from build123d import *

# Parameters (mm, degrees)
F1_DEPTH = 12.7
F2_DEPTH = 6.35
F4_DEPTH = 25.4
F5_DEPTH = 25.4


with BuildPart() as f1:
    # F0 (on Front) → F1 (new body)
    with BuildSketch(Plane.XZ):
        with BuildLine():
            ThreePointArc((38.1, 57.15), (36.240128, 61.640128), (31.75, 63.5))
            Line((31.75, 63.5), (-31.75, 63.5))
            ThreePointArc((-31.75, 63.5), (-36.240128, 61.640128), (-38.1, 57.15))
            Line((-38.1, 57.15), (-38.1, -57.15))
            ThreePointArc((-38.1, -57.15), (-36.240128, -61.640128), (-31.75, -63.5))
            Line((-31.75, -63.5), (31.75, -63.5))
            ThreePointArc((31.75, -63.5), (36.240128, -61.640128), (38.1, -57.15))
            Line((38.1, -57.15), (38.1, 57.15))
        make_face()
        Polygon((22.86, 50.8), (25.4, 50.8), (25.4, 27.760267), (25.4, 23.039733), (25.4, 0), (25.4, -50.8), (-25.4, -50.8), (-25.4, 0), (-25.4, 23.039733), (-25.4, 27.760267), (-25.4, 50.8), (-22.86, 50.8), (-20.32, 50.8), (-17.78, 50.8), (-15.24, 50.8), (-12.7, 50.8), (-10.16, 50.8), (-7.62, 50.8), (-5.08, 50.8), (-2.54, 50.8), (0, 50.8), (2.54, 50.8), (5.08, 50.8), (7.62, 50.8), (10.16, 50.8), (12.7, 50.8), (15.24, 50.8), (17.78, 50.8), (20.32, 50.8), align=None, mode=Mode.SUBTRACT)
    extrude(amount=F1_DEPTH)

    # F0 (on Front) → F2 (join)
    with BuildSketch(Plane.XZ):
        Polygon((22.86, 27.760267), (22.86, 50.8), (20.32, 50.8), (20.32, 27.760267), (17.78, 27.760267), (17.78, 50.8), (15.24, 50.8), (15.24, 27.760267), (12.7, 27.760267), (12.7, 50.8), (10.16, 50.8), (10.16, 27.760267), (7.62, 27.760267), (7.62, 50.8), (5.08, 50.8), (5.08, 27.760267), (2.54, 27.760267), (2.54, 50.8), (0, 50.8), (-2.54, 50.8), (-2.54, 27.760267), (-5.08, 27.760267), (-5.08, 50.8), (-7.62, 50.8), (-7.62, 27.760267), (-10.16, 27.760267), (-10.16, 50.8), (-12.7, 50.8), (-12.7, 27.760267), (-15.24, 27.760267), (-15.24, 50.8), (-17.78, 50.8), (-17.78, 27.760267), (-20.32, 27.760267), (-20.32, 50.8), (-22.86, 50.8), (-22.86, 27.760267), (-25.4, 27.760267), (-25.4, 23.039733), (-22.86, 23.039733), (-22.86, 0), (-20.32, 0), (-20.32, 23.039733), (-17.78, 23.039733), (-17.78, 0), (-15.24, 0), (-15.24, 23.039733), (-12.7, 23.039733), (-12.7, 0), (-10.16, 0), (-10.16, 23.039733), (-7.62, 23.039733), (-7.62, 0), (-5.08, 0), (-5.08, 23.039733), (-2.54, 23.039733), (-2.54, 0), (0, 0), (2.54, 0), (2.54, 23.039733), (5.08, 23.039733), (5.08, 0), (7.62, 0), (7.62, 23.039733), (10.16, 23.039733), (10.16, 0), (12.7, 0), (12.7, 23.039733), (15.24, 23.039733), (15.24, 0), (17.78, 0), (17.78, 23.039733), (20.32, 23.039733), (20.32, 0), (22.86, 0), (22.86, 23.039733), (25.4, 23.039733), (25.4, 27.760267), align=None)
    extrude(amount=F2_DEPTH)

    # F3 (on Right) → F4 (join, through all)
    with BuildSketch(Plane.YZ):
        Polygon((0, -50.8), (0, 0), (-6.35, 0), (-12.7, -50.8), align=None)
    extrude(amount=F4_DEPTH)

    # F4_face (on face) → F5 (join, through all)
    with BuildSketch(Plane(origin=(0, -4.938889, -28.222222), x_dir=(0, 1, 0), z_dir=(-1, 0, 0))):
        Polygon((4.938889, -28.222222), (4.938889, 22.577778), (-7.761111, 22.577778), (-1.411111, -28.222222), align=None)
    extrude(amount=F5_DEPTH)


solid = f1.part
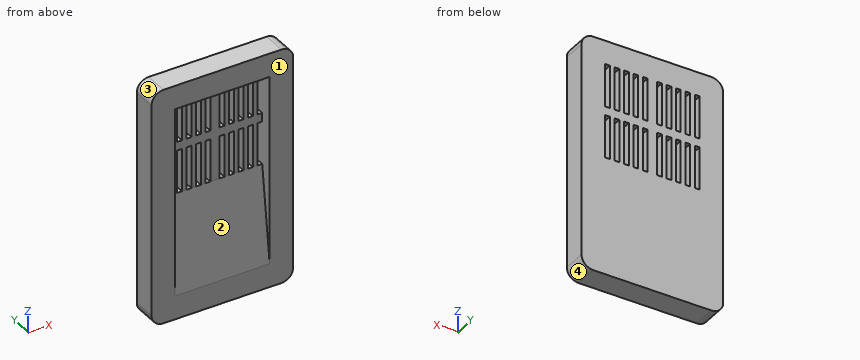
Read the model definition and answer for the solid it produces. Units are mm, in the model's axes. Face numbers are marked on the shaded views. Give positions to 0.01 mm unless a question says otherwise; leave off trailing zeros. Loops run counter-clockwise (first coordinate to the right, second up) from the corner with the lowest first, then second, coordinate; pieces in that order, holes last. Notation, with made-up numbers: (59.5, 13) -> (69.5, 13) arc R34 ccw to (69.5, 47) -> close; hole circle Ø1 at (25, 38). An arc over 180 degrees is marked (long way). Use a Markdown table: item, result.
Q1. Determine the mould class of the marked faces 1, 2, 3 and 4 for opening direction X: pulls with the +X half, pulls with the -X half, needs draft (parallel to the pull), parting line crosses it, or undercut.
Solved:
| item | result |
|---|---|
| face 1 | needs draft |
| face 2 | undercut |
| face 3 | pulls with the -X half |
| face 4 | pulls with the +X half |
Q2. Section B-B, the plane x = 16.5 is taken. Determine the outline of the cut face in (y, z).
Solved:
| item | result |
|---|---|
| outline | (-12.7, -63.5) -> (0, -63.5) -> (0, 63.5) -> (-12.7, 63.5) -> (-12.7, 50.8) -> (-6.35, 50.8) -> (-6.35, 0) -> (-12.7, -50.8) -> close |
Q3. Section A-A, the plane y = -8.75 is taken. Determine the outline of the cut face in (x, z), then the cut area to 3 significant figures.
Solved:
| item | result |
|---|---|
| outline | (-38.1, -57.15) arc R6.35 ccw to (-31.75, -63.5) -> (31.75, -63.5) arc R6.35 ccw to (38.1, -57.15) -> (38.1, 57.15) arc R6.35 ccw to (31.75, 63.5) -> (-31.75, 63.5) arc R6.35 ccw to (-38.1, 57.15) -> close; hole (-25.4, -19.2) -> (25.4, -19.2) -> (25.4, 50.8) -> (-25.4, 50.8) -> close |
| area | 6,090 mm^2 |
Q4. Section D-D, the plane z = 34 is taken. Count the separate pieces of the cut face and the enclosed holes in it, then the cut area to 3 significant figures.
Solved:
| item | result |
|---|---|
| separate pieces | 11 |
| enclosed holes | 0 |
| area | 484 mm^2 |
Q5. Find the intervals of material crossed by line 1 along Z through (x, y) = (-24.5, -1.25); line 2 along X through (y, z) = (-9.5, -2.5); line 3 along Y through (x, z) = (-21.5, 38), in increasing order.
Solved:
| item | result |
|---|---|
| line 1 | z = -63.5 to 0, 23.04 to 27.76, 50.8 to 63.5 |
| line 2 | x = -38.1 to -25.4, 25.4 to 38.1 |
| line 3 | y = -6.35 to 0 |
Q6. Each of these flat-tipped pins is pushed along its axis until it touches: pin 1 (4 mm diameter, centred on x = -6.5, z = 7.5, fed in from -Y); pin 2 (4 mm diameter, centred on x = -0.5, z = -13.5, fed in from -Y). Where does it stop, or does it pass through?
Solved:
| item | result |
|---|---|
| pin 1 | stops at y = -6.35 |
| pin 2 | stops at y = -8.29 |
Q7. Section C-C, the plane z = -24.5 is taken. Determine the outline of the cut face in (x, y).
Solved:
| item | result |
|---|---|
| outline | (-38.1, -12.7) -> (-25.4, -12.7) -> (-25.4, -9.41) -> (25.4, -9.41) -> (25.4, -12.7) -> (38.1, -12.7) -> (38.1, 0) -> (-38.1, 0) -> close |
